Study the drawing (mm; zero at the part's minimum x, y, z) and answer. Coordinates: 2 decimals unless noted, no trailing zeros. Order: outer loops, then holes, each group sorted by start corner. A loop starts at its lowest first (then second) coordinate and runs counter-clockwise, first axis right, second up. Notation, with made-up numbers: M 68,72.5 L 86,72.5 A18 cw 86,102.5 Z; hole C 82.5,-28 d3. An arc over 180 degrees is marked long. Put each result on its own line as item: value.
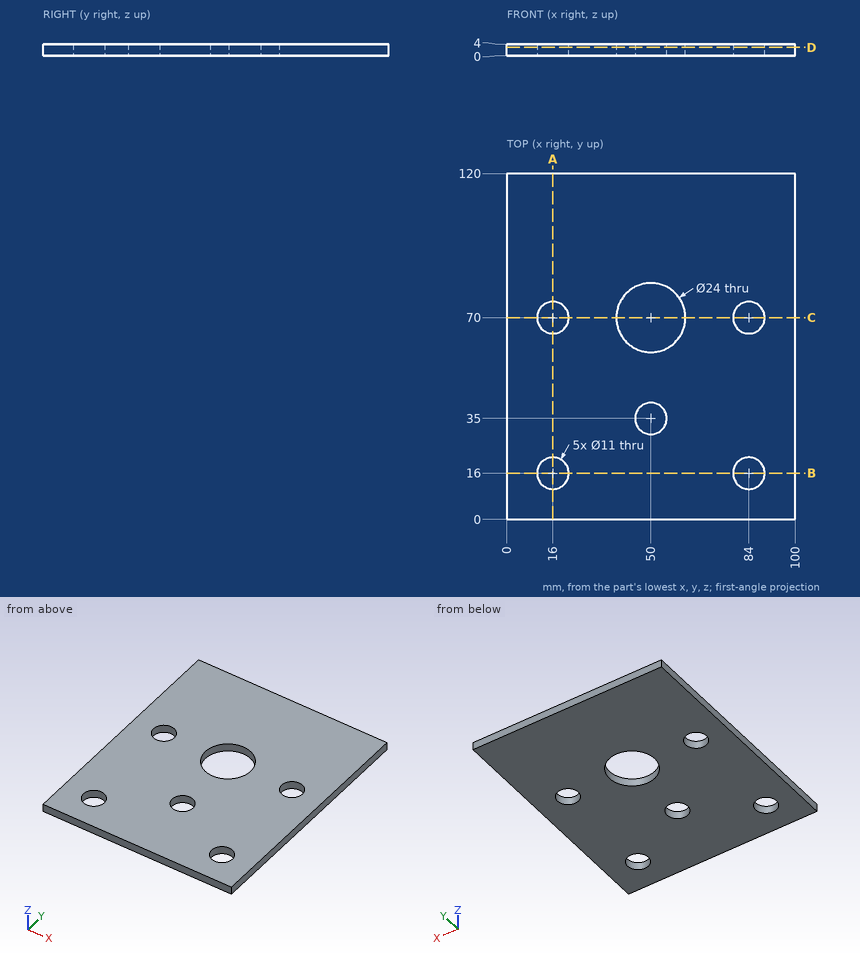
Q1. Find section D-D on z = 2.8. Write down the section's boundary in (x, y).
Answers below:
outline: M 0,0 L 100,0 L 100,120 L 0,120 Z; hole C 16,16 d11; hole C 16,70 d11; hole C 50,70 d24; hole C 50,35 d11; hole C 84,16 d11; hole C 84,70 d11
Q2. Consider line 1 along Y through (x, z) = (84, 2.25); line 2 along Y through (x, z) = (50, 2.3); line 3 along X through (y, z) = (33.5, 1.4). Determine where each line is inside the solid, lowest interval first.
Answers below:
line 1: y = 0 to 10.5, 21.5 to 64.5, 75.5 to 120
line 2: y = 0 to 29.5, 40.5 to 58, 82 to 120
line 3: x = 0 to 44.71, 55.29 to 100
Q3. Given pin 1 (17.5 mm diameter, centred on x = 84, y = 70, fed in from +Z), flat-ended and moving along its own axis, determine where the tip first touches the part or whether it passes through.
Answers below:
pin 1: stops at z = 4
Q4. Find section C-C on y = 70. Write down the section's boundary in (x, z).
Answers below:
outline: M 0,0 L 10.5,0 L 10.5,4 L 0,4 Z; M 21.5,0 L 38,0 L 38,4 L 21.5,4 Z; M 62,0 L 78.5,0 L 78.5,4 L 62,4 Z; M 89.5,0 L 100,0 L 100,4 L 89.5,4 Z
Q5. Find section A-A on x = 16. Write down the section's boundary in (y, z).
Answers below:
outline: M 0,0 L 10.5,0 L 10.5,4 L 0,4 Z; M 21.5,0 L 64.5,0 L 64.5,4 L 21.5,4 Z; M 75.5,0 L 120,0 L 120,4 L 75.5,4 Z
Q6. Find section B-B on y = 16. Write down the section's boundary in (x, z).
Answers below:
outline: M 0,0 L 10.5,0 L 10.5,4 L 0,4 Z; M 21.5,0 L 78.5,0 L 78.5,4 L 21.5,4 Z; M 89.5,0 L 100,0 L 100,4 L 89.5,4 Z
